Part model, mm, in its own coordinate system. A direction names the side the tool comes from. Give positions to 0.01 mm unless a question says otherwise; leave off trailing zeros. Write each loop counter-clockwise with the first axis right and the second up, starting at its lowest first coordinate (ties: lowest second). Pieces come first, ordered by that corner, then holes.
```python
from build123d import *

# Parameters (mm, degrees)
SKETCH1_W           = 88
SKETCH1_H           = 56
BOSS_EXTRUDE1_DEPTH = 18
SKETCH1_3_W         = 38
SKETCH1_3_H         = 12
SKETCH1_3_W_2       = 12
SKETCH1_3_H_2       = 16
SKETCH1_3_H_3       = 28
BOSS_EXTRUDE2_DEPTH = 56
SKETCH4_W           = 161.292605704
SKETCH4_H           = 128.574655565
CUT_EXTRUDE1_DEPTH  = 56


with BuildPart() as part:
    # Sketch1 → Boss-Extrude1 (new body)
    with BuildSketch(Plane(origin=(0, 0, 0), x_dir=(1, 0, 0), z_dir=(0, 1, 0))):
        with Locations((1.76, 28)):
            Rectangle(SKETCH1_W, SKETCH1_H)
    extrude(amount=BOSS_EXTRUDE1_DEPTH)

    # Sketch1_3 → Boss-Extrude2 (add)
    with BuildSketch(Plane(origin=(0, 0, 0), x_dir=(1, 0, 0), z_dir=(0, 1, 0))):
        with Locations((-23.24, 34)):
            Rectangle(SKETCH1_3_W, SKETCH1_3_H)
        with Locations((1.76, 34)):
            Rectangle(SKETCH1_3_W_2, SKETCH1_3_H)
        with Locations((1.76, 48)):
            Rectangle(SKETCH1_3_W_2, SKETCH1_3_H_2)
        with Locations((1.76, 14)):
            Rectangle(SKETCH1_3_W_2, SKETCH1_3_H_3)
        with Locations((26.76, 34)):
            Rectangle(SKETCH1_3_W, SKETCH1_3_H)
    extrude(amount=BOSS_EXTRUDE2_DEPTH)

    # Sketch4 → Cut-Extrude1 (cut)
    with BuildSketch(Plane(origin=(15.253333333, 15.253333333, 15.253333333), x_dir=(0.40824829046386324, 0.40824829046386196, -0.8164965809277265), z_dir=(0.5773502691896268, 0.5773502691896253, 0.5773502691896252))):
        with Locations((33.378380228, 7.240773439)):
            Rectangle(SKETCH4_W, SKETCH4_H)
    extrude(amount=CUT_EXTRUDE1_DEPTH, mode=Mode.SUBTRACT)


solid = part.part
```
1) Saw through at D-D, the plane x = -26. Write the cut outline in (y, z).
Answers follow:
outline: (0, -56) - (18, -56) - (18, -40) - (56, -40) - (56, -28) - (18, -28) - (18, 0) - (0, 0) - close
2) 3-axis set-ups, long thin cutter, end or side, ignore diameter. For faces 1 (the face through (26, 37, -40)), 2 (the face through (-24, 18, -48)), 3 (the face through (22, 18, -14)), 4 (the face through (-6, 56, -37)), 5 (the face through (-4.24, 37, -14)): which of +Z, -Z, +X, -X, +Y, -Y reach the whole face in a straight line?
Answers follow:
face 1: -Z, +X, +Y
face 2: -Z, -X, +Y
face 3: +Z, +X, +Y
face 4: +Z, -Z, +X, -X, +Y
face 5: +Z, -X, +Y
3) Saw through at C-C, the plane y = 41. Write the cut outline in (x, z).
Answers follow:
outline: (-42.24, -40) - (-4.24, -40) - (-4.24, -56) - (7.76, -56) - (7.76, -40) - (44.76, -40) - (32.76, -28) - (7.76, -28) - (7.76, -3) - (4.76, 0) - (-4.24, 0) - (-4.24, -28) - (-42.24, -28) - close
4) Pin check, flat tips, straight feed: pin 1 Ø19 at (x, y) = (-19, 46) entering from -Z; pin 2 Ø5 at (x, y) = (-8.5, 48.5) entering from +Z; pin 3 Ø5 at (x, z) = (-17.5, -45) entering from +Y. Stop position of each tip, or through.
Answers follow:
pin 1: stops at z = -40
pin 2: stops at z = -28
pin 3: stops at y = 18
5) Saw through at A-A, the plane x = 22. Write the cut outline in (y, z), then the cut area to 3 significant figures.
Answers follow:
outline: (0, -56) - (18, -56) - (18, -40) - (56, -40) - (56, -32.24) - (51.76, -28) - (18, -28) - (18, 0) - (0, 0) - close
area: 1,460 mm2
6) Wall check: L1, parallel to Y at x = 32.5, z = -48.5; L2, parallel to Z at x = -23, y = 37; L3, parallel to X at y = 24, z = -17. Give the ranges that are in metal, low to high.
Answers follow:
L1: y = 0 to 18
L2: z = -40 to -28
L3: x = -4.24 to 7.76
7) Saw through at B-B, the plane z = -26. Write the cut outline in (x, y).
Answers follow:
outline: (-42.24, 0) - (45.76, 0) - (45.76, 18) - (7.76, 18) - (7.76, 56) - (-4.24, 56) - (-4.24, 18) - (-42.24, 18) - close
